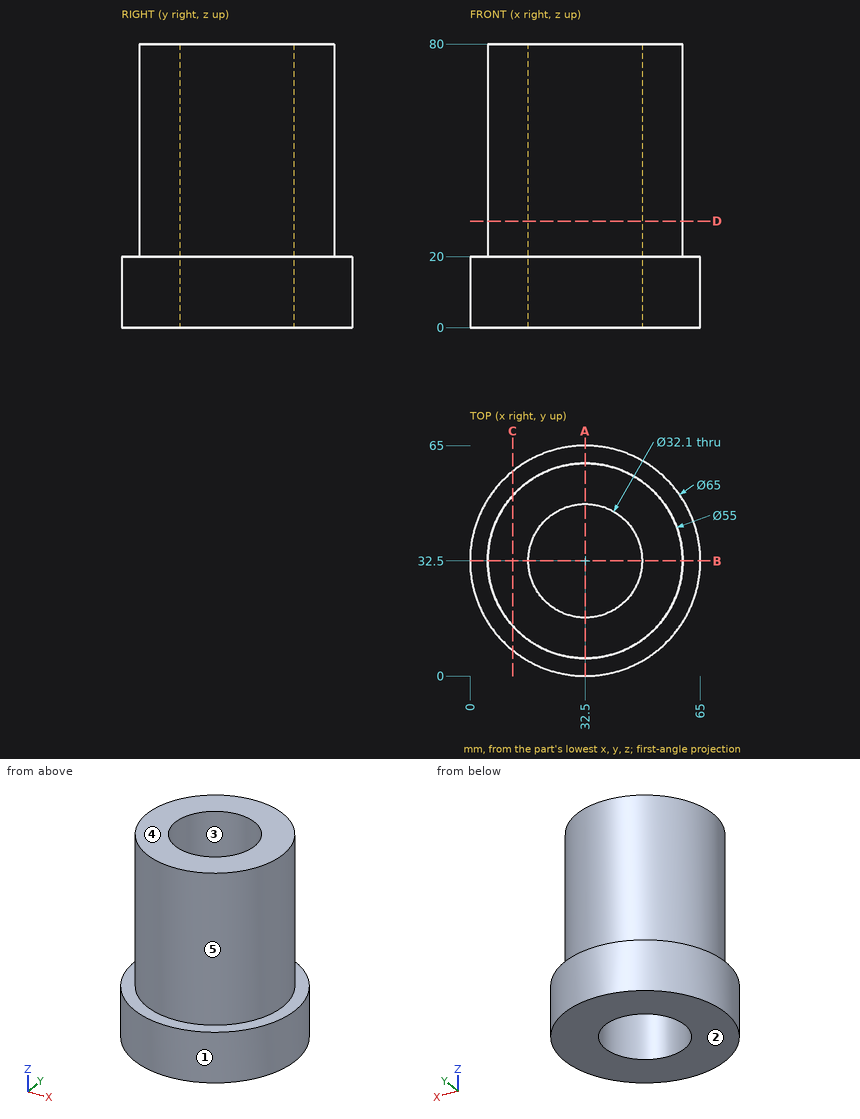
Source: three-view drawing plus pictorial views. Frame: mm from the lowest corner of the part. A direction names the side the tool comes from. Coordinates: 2 decimals unless noted, no trailing zeros. Order: outer loops, then holes, each group sorted by start corner. A loop starts at its lowest first (then second) coordinate and runs counter-clockwise, first axis right, second up. Notation, with made-up numbers: M 42.25,-10.75 L 96.25,-10.75 A17 cw 96.25,5.25 Z; hole C 2.25,84.25 d1. An arc over 180 degrees is marked long. Answer in a Markdown table with one row per item.
(1) Access query for the marked faces 4 and 5. Directions: +Z, -Z, +X, -X, +Y, -Y. A direction counts if a zero-diameter tool reaches every point of the face in a straight line with its end or side. Return the directions, or none.
Numbers:
| item | result |
|---|---|
| face 4 | +Z, +X, -X, +Y, -Y |
| face 5 | +Z |
(2) Section query C-C, the plane x = 12. Output: boundary loops of the cut face in (y, z).
Numbers:
| item | result |
|---|---|
| outline | M 7.28,0 L 57.72,0 L 57.72,20 L 50.83,20 L 50.83,80 L 14.17,80 L 14.17,20 L 7.28,20 Z |
(3) Contact query for flat-ended pins moving along their axis: pin 1 Ø1 at (y, z) = (25, 49) entering from +X; pin 2 Ø12 at (x, z) = (53.5, 21.5) entering from +Y; pin 3 Ø3 at (y, z) = (43, 53.5) entering from -X. Output: stop coordinate, or through.
Numbers:
| item | result |
|---|---|
| pin 1 | stops at x = 59.09 |
| pin 2 | stops at y = 61.23 |
| pin 3 | stops at x = 6.51 |
(4) Section query D-D, the plane z = 30. Output: boundary loops of the cut face in (x, y).
Numbers:
| item | result |
|---|---|
| outline | C 32.5,32.5 d55; hole C 32.5,32.5 d32.1 |
(5) Section query A-A, the plane x = 32.5. Output: boundary loops of the cut face in (y, z), plus the area to 3 significant figures.
Numbers:
| item | result |
|---|---|
| outline | M 0,0 L 16.45,0 L 16.45,80 L 5,80 L 5,20 L 0,20 Z; M 48.55,0 L 65,0 L 65,20 L 60,20 L 60,80 L 48.55,80 Z |
| area | 2,030 mm^2 |
(6) Draft query along Y for the marked faces 1, 2 and 3. Return one class per face: pulls with the +Y half, pulls with the -Y half, needs draft (parallel to the pull), parting line crosses it, or undercut.
Numbers:
| item | result |
|---|---|
| face 1 | parting line crosses it |
| face 2 | needs draft |
| face 3 | undercut |
(7) Material intervals for line 1 (Y direction, x = 32.5, z = 53.5); line 2 (X direction, y = 32, z = 48); line 3 (Z direction, x = 43, y = 59.5), sorted ascending. Write a range as [from, to].
Numbers:
| item | result |
|---|---|
| line 1 | y = [5, 16.45], [48.55, 60] |
| line 2 | x = [5, 16.46], [48.54, 60] |
| line 3 | z = [0, 20] |
